Model file for the job. Use its own axes, mm. Face numbers are marked on the shaded views. Give positions to 0.01 mm unless a question says otherwise; leave off trailing zeros. Loops run counter-clockwise (first coordinate to the right, second up) from the corner with the lowest first, then second, coordinate; pieces in that order, holes last. Notation, with made-up numbers: M -30.75,-36.5 L -16.75,-36.5 A33 ccw -16.75,-8.5 Z; hole C 24.5,70 d4. An arc over 180 degrees is marked long. Use CSV: the item, a comma, the result in double quotes. Start each with the question number.
(1) Flat gauge pins, fed straight in: P1, Ø6, axis at x = 7, z = -2.5, coming from the +Y side; P2, Ø0.6, axis at x = 9, z = -23, coming from the +Y side; P3, Ø6, axis at x = -12, z = -36.5, coming from the -Y side. Where does each tip first touch, or does it go through?
(2) Slice it at B-B on y = 4. List the corners of the cut face in (x, z), and give its area (3 significant figures).
(3) Slice it at A-A on z = -12.5. List the corners of the cut face in (x, y), and give its area (3 significant figures).
(4) Wall check: line 1 along X through (y, z) = (4.5, -12.5); line 2 along X through (y, z) = (-5.25, 39); line 3 along Y through (x, z) = (18.5, 12.5). Give the ranges that are in metal, low to high. Write a range as from..to.
(5) Slice it at C-C on x = 15.5. List the corners of the cut face in (y, z).
(6) Two-plate mould, pull along X, no slides. Class the marked faces 1, 2 and 3: pulls with the +X half, pulls with the -X half, needs draft (parallel to the pull), parting line crosses it, or undercut.
(7) Slice it at D-D on y = -5.5. List the corners of the cut face in (x, z), and give its area (3 significant figures).
```python
from build123d import *

# Parameters (mm, degrees)
F0_R          = 9
F1_DEPTH      = 68
F2_W          = 40
F2_H          = 5
F3_DEPTH      = 68
F3_DEPTH_BACK = 68


with BuildPart() as f1:
    # F0 (on Top) → F1 (new body, symmetric)
    with BuildSketch(Plane.XY):
        with Locations((-18, 0)):
            Circle(F0_R)
    extrude(amount=F1_DEPTH, both=True)



with BuildPart() as f1b:
    # F0 (on Top) → F1, piece 2 (new body, symmetric)
    with BuildSketch(Plane.XY):
        with BuildLine():
            ThreePointArc((27, 0), (18, 9), (9, 0))
            ThreePointArc((9, 0), (18, -9), (27, 0))
        make_face()
    extrude(amount=F1_DEPTH, both=True)


with BuildPart() as f1c:
    # F0 (on Top) → F1, piece 3 (new body, symmetric)
    with BuildSketch(Plane.XY):
        with BuildLine():
            ThreePointArc((9, 0), (0, 9), (-9, 0))
            ThreePointArc((-9, 0), (0, -9), (9, 0))
        make_face()
    extrude(amount=F1_DEPTH, both=True)


with BuildPart() as f1_1:
    add(f1.part)

    add(f1b.part)  # F3 merges F1b

    add(f1c.part)  # F3 merges F1c
    # F2 (on Top) → F3 (join, two sides)
    with BuildSketch(Plane.XY) as f3_sk:
        Rectangle(F2_W, F2_H)
    extrude(amount=F3_DEPTH)
    extrude(f3_sk.sketch, amount=-F3_DEPTH_BACK)


solid = f1_1.part
```
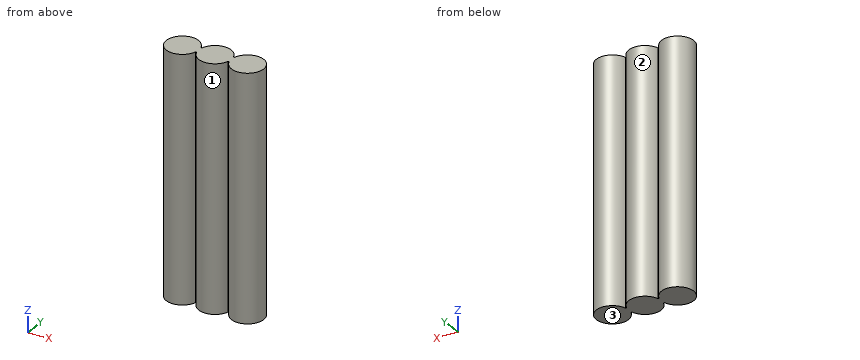
Reply:
1,P1,"stops at y = 8.06"
1,P2,"stops at y = 2.5"
1,P3,"stops at y = -8.49"
2,outline,"M -26.06,-68 L -9.94,-68 L -9.94,68 L -26.06,68 Z; M -8.06,-68 L 8.06,-68 L 8.06,68 L -8.06,68 Z; M 9.94,-68 L 26.06,-68 L 26.06,68 L 9.94,68 Z"
2,area,"6,580 mm^2"
3,outline,"M -9.35,-2.5 L -8.65,-2.5 A9 ccw 8.65,-2.5 L 9.35,-2.5 A9 ccw long 9.35,2.5 L 8.65,2.5 A9 ccw -8.65,2.5 L -9.35,2.5 A9 ccw long Z"
3,area,"766 mm^2"
4,line 1,"x = -25.79..-10.21, -7.79..7.79, 10.21..25.79"
4,line 2,"x = -25.31..-10.69, -7.31..7.31, 10.69..25.31"
4,line 3,"y = -8.99..8.99"
5,outline,"M -8.65,-68 L 8.65,-68 L 8.65,68 L -8.65,68 Z"
6,face 1,"undercut"
6,face 2,"undercut"
6,face 3,"needs draft"
7,outline,"M -25.12,-68 L -10.88,-68 L -10.88,68 L -25.12,68 Z; M -7.12,-68 L 7.12,-68 L 7.12,68 L -7.12,68 Z; M 10.88,-68 L 25.12,-68 L 25.12,68 L 10.88,68 Z"
7,area,"5,810 mm^2"
